Read the model definition and answer for the solid it produces. Units are mm, in the model's axes. Round coordinates to 2 decimals unless told otherwise and drop trailing zeros. Loops run counter-clockwise (first coordinate to the right, second up) from the corner with the lowest first, then second, coordinate; pieces in that order, holes last. Notation, with made-up numbers: (14, 71.5) -> (37, 71.5) arc R27 ccw to (37, 88.5) -> close; hole circle Ø2 at (80.5, -11). An arc over 180 degrees is marked (long way). Put each result on its own line as item: value.
from build123d import *

# Parameters (mm, degrees)
CYLINDER_R     = 2
CYLINDER_DEPTH = 15
ARRAY_X_COUNT  = 2
ARRAY_X_PITCH  = 35
BOX_W          = 44
BOX_H          = 12
BOX_DEPTH      = 8
FILLET003_R    = 3


with BuildPart() as array:
    # Cylinder → Cylinder (new body)
    with BuildSketch(Plane(origin=(-17.5, 0, -10), x_dir=(1, 0, 0), z_dir=(0, 0, 1))):
        Circle(CYLINDER_R)
    extrude(amount=CYLINDER_DEPTH)

    # Array X: Array ×2


with BuildPart() as array_1:
    add(array.part)
    with Locations(*[(i * ARRAY_X_PITCH, 0, 0) for i in range(1, ARRAY_X_COUNT)]):
        add(array.part)


with BuildPart() as cut:
    # Box → Box (new body)
    with BuildSketch(Plane(origin=(-22, -6, -8), x_dir=(1, 0, 0), z_dir=(0, 0, 1))):
        with Locations((22, 6)):
            Rectangle(BOX_W, BOX_H)
    extrude(amount=BOX_DEPTH)

    # Fillet003
    fillet003_edges = [cut.edges().sort_by_distance(p)[0] for p in [
        (-22, -6, -4),
        (-22, 6, -4),
        (22, -6, -4),
        (22, 6, -4),
    ]]
    fillet(fillet003_edges, radius=FILLET003_R)

    # Cut: cut Array
    add(array_1.part, mode=Mode.SUBTRACT)


solid = cut.part
Item 1: The part is cut by section C-C (x = 17.5). Determine the outline of the cut face in (y, z), then the cut area to 3 significant figures.
Derived:
outline: (-6, -8) -> (-2, -8) -> (-2, 0) -> (-6, 0) -> close; (2, -8) -> (6, -8) -> (6, 0) -> (2, 0) -> close
area: 64.0 mm^2
Item 2: The part is cut by section D-D (y = -5). Determine the outline of the cut face in (x, z).
Derived:
outline: (-21.24, -8) -> (21.24, -8) -> (21.24, 0) -> (-21.24, 0) -> close
Item 3: Find the intervals of material crossed by line 1 along X through (y, z) = (0, -5.25); line 2 along Y through (x, z) = (-17.5, -1.75); line 3 along X through (y, z) = (0.5, -0.75), in increasing order.
Derived:
line 1: x = -22 to -19.5, -15.5 to 15.5, 19.5 to 22
line 2: y = -6 to -2, 2 to 6
line 3: x = -22 to -19.44, -15.56 to 15.56, 19.44 to 22
Item 4: For a pull along Y with two mould halves and no side action, classify faces 1 (the flat face through (0, 0, 0)), 2 (the flat face through (0, -6, -4)), 3 (the flat face through (0, 6, -4)), 4 (the cylindrical face through (-19.1, -1.2, -4.1)) as pulls with the +Y half, pulls with the -Y half, needs draft (parallel to the pull), parting line crosses it, or undercut.
Derived:
face 1: needs draft
face 2: pulls with the -Y half
face 3: pulls with the +Y half
face 4: undercut
Item 5: A flat-ended cylindrical pin translates along its axis: pin 1 Ø6 at (x, y) = (4.5, -0.5) entering from +Z. Find the tip coordinate at first contact, or state that the pin passes through.
Derived:
pin 1: stops at z = 0
Item 6: The part is cut by section A-A (y = 0). Determine the outline of the cut face in (x, z).
Derived:
outline: (-22, -8) -> (-19.5, -8) -> (-19.5, 0) -> (-22, 0) -> close; (-15.5, -8) -> (15.5, -8) -> (15.5, 0) -> (-15.5, 0) -> close; (19.5, -8) -> (22, -8) -> (22, 0) -> (19.5, 0) -> close
Item 7: The part is cut by section B-B (z = -3.5). Determine the outline of the cut face in (x, y), then the cut area to 3 significant figures.
Derived:
outline: (-22, -3) arc R3 ccw to (-19, -6) -> (19, -6) arc R3 ccw to (22, -3) -> (22, 3) arc R3 ccw to (19, 6) -> (-19, 6) arc R3 ccw to (-22, 3) -> close; hole circle Ø4 at (-17.5, 0); hole circle Ø4 at (17.5, 0)
area: 495 mm^2
